from build123d import *

# Parameters (mm, degrees)
BOSS_EXTRUDE1_DEPTH = 70
SKETCH2_R           = 130
BOSS_EXTRUDE2_DEPTH = 100
SKETCH5_R           = 10
CUT_EXTRUDE1_DEPTH  = 324.960703978
SKETCH6_R           = 100
CUT_EXTRUDE2_DEPTH  = 90


with BuildPart() as part:
    # Sketch1 → Boss-Extrude1 (new body)
    with BuildSketch(Plane(origin=(0, 0, 0), x_dir=(1, 0, 0), z_dir=(0, 1, 0))):
        with BuildLine():
            Line((-85.450778727, 179.708800959), (96.227625611, 179.708800959))
            ThreePointArc((96.227625611, 179.708800959), (102.682597854, 182.071174801), (106.087758582, 188.042134293))
            ThreePointArc((106.087758582, 188.042134293), (189.081994137, 216.651233118), (168.212109643, 131.381240787))
            ThreePointArc((168.212109643, 131.381240787), (162.850707457, 127.812966963), (160.776846883, 121.715728753))
            Line((160.776846883, 121.715728753), (160.776846883, -121.715728753))
            ThreePointArc((160.776846883, -121.715728753), (162.850707457, -127.812966963), (168.212109643, -131.381240787))
            ThreePointArc((168.212109643, -131.381240787), (189.081994137, -216.651233118), (106.087758582, -188.042134293))
            ThreePointArc((106.087758582, -188.042134293), (102.682597854, -182.071174801), (96.227625611, -179.708800959))
            Line((96.227625611, -179.708800959), (-85.450778727, -179.708800959))
            ThreePointArc((-85.450778727, -179.708800959), (-91.905750971, -182.071174801), (-95.310911699, -188.042134293))
            ThreePointArc((-95.310911699, -188.042134293), (-178.305147254, -216.651233118), (-157.43526276, -131.381240787))
            ThreePointArc((-157.43526276, -131.381240787), (-152.073860574, -127.812966963), (-150, -121.715728753))
            Line((-150, -121.715728753), (-150, 121.715728753))
            ThreePointArc((-150, 121.715728753), (-152.073860574, 127.812966963), (-157.43526276, 131.381240787))
            ThreePointArc((-157.43526276, 131.381240787), (-178.305147254, 216.651233118), (-95.310911699, 188.042134293))
            ThreePointArc((-95.310911699, 188.042134293), (-91.905750971, 182.071174801), (-85.450778727, 179.708800959))
        make_face()
    extrude(amount=BOSS_EXTRUDE1_DEPTH)

    # Sketch2 → Boss-Extrude2 (add)
    with BuildSketch(Plane(origin=(0, 70, 0), x_dir=(1, 0, 0), z_dir=(0, 1, 0))):
        with Locations(Location((0, 0, 0), (0, 0, 90))):
            Circle(SKETCH2_R)
    extrude(amount=BOSS_EXTRUDE2_DEPTH)

    # Sketch5 → Cut-Extrude1 (cut, through all)
    with BuildSketch(Plane(origin=(0, 70, 0), x_dir=(1, 0, 0), z_dir=(0, 1, 0))):
        with Locations(Location((-144.611576558, -179.708800959, 0), (0, 0, 270))):
            Circle(SKETCH5_R)
        with Locations(Location((-144.611576558, 179.708800959, 0), (0, 0, 270))):
            Circle(SKETCH5_R)
        with Locations(Location((155.388423442, -179.708800959, 0), (0, 0, 270))):
            Circle(SKETCH5_R)
        with Locations(Location((155.388423442, 179.708800959, 0), (0, 0, 270))):
            Circle(SKETCH5_R)
    extrude(amount=-CUT_EXTRUDE1_DEPTH, mode=Mode.SUBTRACT)

    # Sketch6 → Cut-Extrude2 (cut)
    with BuildSketch(Plane(origin=(0, 170, 0), x_dir=(1, 0, 0), z_dir=(0, 1, 0))):
        with Locations(Location((0, 0, 0), (0, 0, 270))):
            Circle(SKETCH6_R)
    extrude(amount=-CUT_EXTRUDE2_DEPTH, mode=Mode.SUBTRACT)


solid = part.part
Can you work these out from the model? Positions are in its coordinate system, mm. A direction names the side the tool comes from. Coordinates: 2 decimals unless noted, no trailing zeros. Loops run counter-clockwise (first coordinate to the right, second up) from the corner with the lowest first, then second, coordinate; pieces in that order, holes last. Notation, with made-up numbers: M 42.25,83.25 L 99.25,83.25 A14 ccw 99.25,102.25 Z; hole C -40,43.25 d3. An arc over 180 degrees is marked long. Answer as CSV lines item,"result". Start each with the question number.
1. If I drill on probe 1 along X at (y, z) = (103, 0); probe 2 along Z at (x, y) = (50, 62); probe 3 along Y at (x, z) = (119.5, -178), over which ranges is the centre line in solid material (lowest first)? Write a range as [from, to].
2. Thinking about a two-plate mould opening in X: for faces 6 (the face through (142, 70, -3)), 7 (the face through (-39.048, 119.3, -123.997)), 8 (the face through (1, 80, -1)), which applies, +X half, -X half, draft (parallel to the pull), parting line (faces both ways), or undercut?
3. Suppose I cut it at A-A, the plane x = 0. List the corners of the cut face in (y, z) for me.
4. Suppose I cut it at D-D, the plane y = 131. List the corners of the cut face in (x, z) for me, plus the area to 3 significant figures.
5. Suppose I cut it at C-C, the plane y = 18.5. List the corners of the cut face in (x, z) for me.
6. For faces 1 (the face through (-152.02, 34.51, -127.74)), 2 (the face through (4, 35, -179.709)), 3 (the face through (30.04, 125.63, 95.38)), 4 (the face through (7, 35, 179.709)), 5 (the face through (163, 35, 128)), which set-ups out of +Z, -Z, +X, -X, +Y, -Y let a thin tool reach every point of the face, with its end or its side?
7. Suppose I cut it at B-B, the plane z = 0. List the corners of the cut face in (x, y) for me.
8. For pin 1 Ø4 at (x, y) = (-110, 34.5) entering from +Z; pin 2 Ø4 at (x, y) = (-34.5, 45.5) entering from +Z; pin 3 Ø8 at (y, z) = (44.5, -88) entering from -X; pin 4 Ø16 at (x, z) = (155.39, 179.71) entering from +Y, each with a flat end and sliding along its axis, tell me the tip position at first contact or that it passes through.
Output:
1,probe 1,"x = [-130, -100], [100, 130]"
1,probe 2,"z = [-179.71, 179.71]"
1,probe 3,"y = [0, 70]"
2,face 6,"draft"
2,face 7,"parting line"
2,face 8,"undercut"
3,outline,"M 0,-179.71 L 70,-179.71 L 70,-130 L 170,-130 L 170,-100 L 80,-100 L 80,100 L 170,100 L 170,130 L 70,130 L 70,179.71 L 0,179.71 Z"
4,outline,"C 0,0 d260; hole C 0,0 d200"
4,area,"21,700 mm^2"
5,outline,"M -157.44,-131.38 A50 ccw long -95.31,-188.04 A10 cw -85.45,-179.71 L 96.23,-179.71 A10 cw 106.09,-188.04 A50 ccw long 168.21,-131.38 A10 cw 160.78,-121.72 L 160.78,121.72 A10 cw 168.21,131.38 A50 ccw long 106.09,188.04 A10 cw 96.23,179.71 L -85.45,179.71 A10 cw -95.31,188.04 A50 ccw long -157.44,131.38 A10 cw -150,121.72 L -150,-121.72 A10 cw Z; hole C -144.61,-179.71 d20; hole C -144.61,179.71 d20; hole C 155.39,-179.71 d20; hole C 155.39,179.71 d20"
6,face 1,"-X, +Y, -Y"
6,face 2,"-Z, +Y, -Y"
6,face 3,"+Y"
6,face 4,"+Z, +Y, -Y"
6,face 5,"+X, +Y, -Y"
7,outline,"M -150,0 L 160.78,0 L 160.78,70 L 130,70 L 130,170 L 100,170 L 100,80 L -100,80 L -100,170 L -130,170 L -130,70 L -150,70 Z"
8,pin 1,"stops at z = 217.61"
8,pin 2,"stops at z = 179.71"
8,pin 3,"stops at x = -150"
8,pin 4,"passes through"
